Part model, mm, in its own coordinate system. Face numbers are marked on the shaded views. Coordinates: 2 decimals unless noted, no trailing zeros. Loops run counter-clockwise (first coordinate to the right, second up) from the corner with the lowest first, then second, coordinate; pieces in that order, holes last. Notation, with made-up numbers: M 81.5,6 L 116.5,6 A16 cw 116.5,29 Z; hole C 23.25,-29 d1. An arc over 180 degrees is marked long. Use a Markdown table: item, result. Add a question column.
1) Band-saw the part on C-C (x = 224.5). List the corners of the cut face in (y, z), plus the area to 3 significant figures.
2) Wall check: probe 1 along Y at (x, z) = (26.5, -12.5); probe 2 along Y at (x, z) = (26.5, -9.25); probe 3 along Z at (x, y) = (249, 51.5). Give the ranges that are in metal, low to high. Write a range as from..to.
3) Band-saw the part on B-B (x = 65). List the corners of the cut face in (y, z).
4) Pull direction Y, two halves, no side cores. Call the marked faces 1 and 2: released by +Y, released by -Y, zero draft, split by the parting line, or undercut.
5) Pin check, flat tips, straight feed: pin 1 Ø0.8 at (x, z) = (112.5, -14.5) entering from -Y; pin 2 Ø0.8 at (x, z) = (140, -14.5) entering from +Y; pin 3 Ø1.4 at (x, y) = (165, 69) entering from -Z; pin 4 Ø1 at (y, z) = (60, -11.5) entering from -X. Stop position of each tip, or through.
6) Band-saw the part on A-A (z = -11.75). List the corners of the cut face in (x, y), plus the area to 3 significant figures.
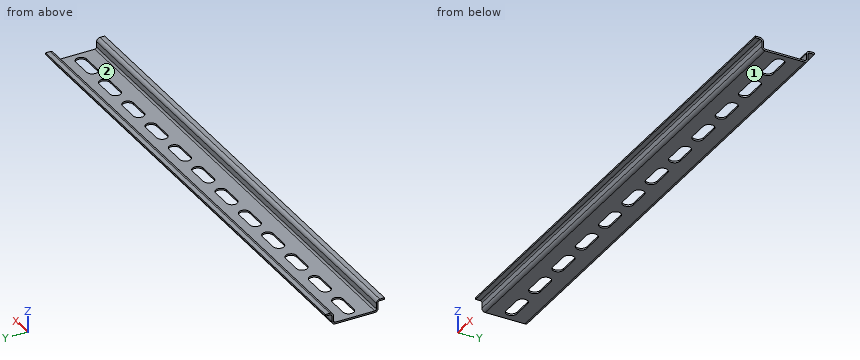
Autodesk Inventor part; units mm, degrees
ref_plane "YZ Plane" through (0, 0, 0) normal (1, 0, 0) x (0, 1, 0)
ref_plane "XZ Plane" through (0, 0, 0) normal (0, 1, 0) x (-1, 0, 0)
ref_plane "XY Plane" through (0, 0, 0) normal (0, 0, 1) x (1, 0, 0)
sketch "Sketch1" plane through (0, 0, 0) normal (1, 0, 0) x (0, 1, 0)
  line L0 (41.284, -14.8819) -> (64.684, -14.8819)
  line L1 (64.684, -13.8819) -> (41.284, -13.8819)
  line L2 (67.684, -8.5819) -> (70.484, -8.5819)
  line L3 (70.484, -8.5819) -> (70.484, -7.5819)
  line L4 (70.484, -7.5819) -> (67.684, -7.5819)
  line L5 (-1817770.1114, -20.3632) -> (-1817770.1114, -8.5819)
  line L6 (38.284, -7.5819) -> (35.484, -7.5819)
  line L7 (35.484, -7.5819) -> (35.484, -8.5819)
  line L8 (35.484, -8.5819) -> (38.284, -8.5819)
  line L9 (40.284, -9.5819) -> (40.284, -12.8819)
  arc A0 (67.684, -8.5819) -> (66.684, -9.5819) centre (67.684, -9.5819) ccw
  arc A1 (64.684, -13.8819) -> (65.684, -12.8819) centre (64.684, -12.8819) ccw
  arc A2 (40.284, -12.8819) -> (41.284, -13.8819) centre (41.284, -12.8819) ccw
  arc A3 (39.284, -9.5819) -> (38.284, -8.5819) centre (38.284, -9.5819) ccw
  arc A4 (40.284, -9.5819) -> (38.284, -7.5819) centre (38.284, -9.5819) ccw
  arc A5 (39.284, -12.8819) -> (41.284, -14.8819) centre (41.284, -12.8819) ccw
  line L10 (39.284, -9.5819) -> (39.284, -12.8819)
  arc A6 (67.684, -7.5819) -> (65.684, -9.5819) centre (67.684, -9.5819) ccw
  arc A7 (64.684, -14.8819) -> (66.684, -12.8819) centre (64.684, -12.8819) ccw
  line L11 (66.684, -9.5819) -> (66.684, -12.8819)
  line L12 (65.684, -9.5819) -> (65.684, -12.8819)
  line L13 (52.984, -4.8951) -> (52.984, -40.6352) construction
  line L14 (-285.558, -25.9225) -> (179.442, -25.9225)
  line L15 (179.442, -25.9225) -> (179.442, -22.9225)
  line L16 (-285.558, -22.9225) -> (179.442, -22.9225)
  line L17 (-285.558, -25.9225) -> (-285.558, -22.9225)
  point P0 (0, 0)
  point P1 (40.284, -11.2319)
  dimension "d0" = 1
  dimension "d1" = 1
  dimension "d5" = 35
  dimension "d8" = 7.3
  dimension "d9" = 1
  dimension "d10" = 1
  dimension "d11" = 2
  dimension "d12" = 2
  dimension "d13" = 12.7
  dimension "d15" = 12.7
  dimension "d16" = 4.8
  dimension "d17" = 4.8
  dimension "d20" = 1
  dimension "d21" = 1
  dimension "d22" = 2
extrude "Extrusion1" add sketch "Sketch1" along normal blind 300 contours A5 L10 A3 L8 L7 L6 A4 L9 A2 L1 A1 L12 A6 L4 L3 L2 A0 L11 A7 L0
sketch "Sketch2" plane through (0, 41.284, -13.8819) normal (0, 0, 1) x (1, 0, 0)
  line L0 (3.6, 11.7) -> (21.6, 11.7) construction
  line L1 (6.8, 8.5) -> (18.4, 8.5)
  line L2 (18.4, 14.9) -> (6.8, 14.9)
  arc A0 (6.8, 14.9) -> (6.8, 8.5) centre (6.8, 11.7) ccw
  arc A1 (18.4, 8.5) -> (18.4, 14.9) centre (18.4, 11.7) ccw
  line L3 (0, 29.2) -> (300, 29.2)
  line L4 (0, -5.8) -> (300, -5.8)
  line L5 (0, 23.4) -> (0, 0)
  arc A2 (31.8, 14.9) -> (31.8, 8.5) centre (31.8, 11.7) ccw
  line L6 (31.8, 8.5) -> (43.4, 8.5)
  arc A3 (43.4, 8.5) -> (43.4, 14.9) centre (43.4, 11.7) ccw
  line L7 (43.4, 14.9) -> (31.8, 14.9)
  arc A4 (56.8, 14.9) -> (56.8, 8.5) centre (56.8, 11.7) ccw
  line L8 (56.8, 8.5) -> (68.4, 8.5)
  arc A5 (68.4, 8.5) -> (68.4, 14.9) centre (68.4, 11.7) ccw
  line L9 (68.4, 14.9) -> (56.8, 14.9)
  arc A6 (81.8, 14.9) -> (81.8, 8.5) centre (81.8, 11.7) ccw
  line L10 (81.8, 8.5) -> (93.4, 8.5)
  arc A7 (93.4, 8.5) -> (93.4, 14.9) centre (93.4, 11.7) ccw
  line L11 (93.4, 14.9) -> (81.8, 14.9)
  arc A8 (106.8, 14.9) -> (106.8, 8.5) centre (106.8, 11.7) ccw
  line L12 (106.8, 8.5) -> (118.4, 8.5)
  arc A9 (118.4, 8.5) -> (118.4, 14.9) centre (118.4, 11.7) ccw
  line L13 (118.4, 14.9) -> (106.8, 14.9)
  arc A10 (131.8, 14.9) -> (131.8, 8.5) centre (131.8, 11.7) ccw
  line L14 (131.8, 8.5) -> (143.4, 8.5)
  arc A11 (143.4, 8.5) -> (143.4, 14.9) centre (143.4, 11.7) ccw
  line L15 (143.4, 14.9) -> (131.8, 14.9)
  arc A12 (156.8, 14.9) -> (156.8, 8.5) centre (156.8, 11.7) ccw
  line L16 (156.8, 8.5) -> (168.4, 8.5)
  arc A13 (168.4, 8.5) -> (168.4, 14.9) centre (168.4, 11.7) ccw
  line L17 (168.4, 14.9) -> (156.8, 14.9)
  arc A14 (181.8, 14.9) -> (181.8, 8.5) centre (181.8, 11.7) ccw
  line L18 (181.8, 8.5) -> (193.4, 8.5)
  arc A15 (193.4, 8.5) -> (193.4, 14.9) centre (193.4, 11.7) ccw
  line L19 (193.4, 14.9) -> (181.8, 14.9)
  line L20 (0, 0) -> (300, 0)
  line L21 (0, 24.4) -> (300, 24.4)
  line L22 (0, -1) -> (300, -1)
  arc A16 (206.8, 14.9) -> (206.8, 8.5) centre (206.8, 11.7) ccw
  line L23 (218.4, 14.9) -> (206.8, 14.9)
  arc A17 (218.4, 8.5) -> (218.4, 14.9) centre (218.4, 11.7) ccw
  line L24 (206.8, 8.5) -> (218.4, 8.5)
  arc A18 (231.8, 14.9) -> (231.8, 8.5) centre (231.8, 11.7) ccw
  line L25 (243.4, 14.9) -> (231.8, 14.9)
  arc A19 (243.4, 8.5) -> (243.4, 14.9) centre (243.4, 11.7) ccw
  line L26 (231.8, 8.5) -> (243.4, 8.5)
  arc A20 (256.8, 14.9) -> (256.8, 8.5) centre (256.8, 11.7) ccw
  line L27 (268.4, 14.9) -> (256.8, 14.9)
  arc A21 (268.4, 8.5) -> (268.4, 14.9) centre (268.4, 11.7) ccw
  line L28 (256.8, 8.5) -> (268.4, 8.5)
  arc A22 (281.8, 14.9) -> (281.8, 8.5) centre (281.8, 11.7) ccw
  line L29 (293.4, 14.9) -> (281.8, 14.9)
  arc A23 (293.4, 8.5) -> (293.4, 14.9) centre (293.4, 11.7) ccw
  line L30 (281.8, 8.5) -> (293.4, 8.5)
  point P0 (0, -41.284)
  point P1 (12.6, 11.7)
  point P2 (28.6, 11.7)
  point P3 (46.6, 11.7)
  point P4 (53.6, 11.7)
  point P5 (71.6, 11.7)
  point P6 (78.6, 11.7)
  point P7 (96.6, 11.7)
  point P8 (103.6, 11.7)
  point P9 (121.6, 11.7)
  point P10 (128.6, 11.7)
  point P11 (146.6, 11.7)
  point P12 (153.6, 11.7)
  point P13 (171.6, 11.7)
  point P14 (178.6, 11.7)
  point P15 (196.6, 11.7)
  point P16 (28.6, 11.7)
  point P17 (203.6, 11.7)
  point P18 (221.6, 11.7)
  point P19 (228.6, 11.7)
  point P20 (246.6, 11.7)
  point P21 (253.6, 11.7)
  point P22 (271.6, 11.7)
  point P23 (278.6, 11.7)
  point P24 (296.6, 11.7)
  dimension "d26" = 18
  dimension "d33" = 25
  dimension "d46" = 3.6
  dimension "d47" = 17.5
  dimension "d48" = 17.5
  dimension "d51" = 25
extrude "Extrusion2" cut sketch "Sketch2" against normal blind 25
sketch "Sketch3" plane through (0, 41.284, -13.8819) normal (0, 0, 1) x (1, 0, 0)
  line L0 (110, 34.2) -> (302, 34.2)
  line L1 (302, 34.2) -> (302, -10.8)
  line L2 (302, -10.8) -> (110, -10.8)
  line L3 (110, -10.8) -> (110, 34.2)
  line L4 (0, 23.4) -> (0, 0)
  line L5 (300, 23.4) -> (300, 0)
  line L6 (0, -5.8) -> (300, -5.8)
  line L7 (0, 29.2) -> (300, 29.2)
  point P0 (0, -41.284)
  dimension "d56" = 110
  dimension "d57" = 2
  dimension "d58" = 5
  dimension "d59" = 5
equation "\"d39\" = d33"
properties part number "DIN-rail"
Entries:
| question | item | result |
|---|---|---|
| 1 | outline | M 35.48,-8.58 L 38.28,-8.58 A1 cw 39.28,-9.58 L 39.28,-12.88 A2 ccw 41.28,-14.88 L 64.68,-14.88 A2 ccw 66.68,-12.88 L 66.68,-9.58 A1 cw 67.68,-8.58 L 70.48,-8.58 L 70.48,-7.58 L 67.68,-7.58 A2 ccw 65.68,-9.58 L 65.68,-12.88 A1 cw 64.68,-13.88 L 41.28,-13.88 A1 cw 40.28,-12.88 L 40.28,-9.58 A2 ccw 38.28,-7.58 L 35.48,-7.58 Z |
| 1 | area | 45.0 mm2 |
| 2 | probe 1 | 39.28..40.28, 65.68..66.68 |
| 2 | probe 2 | 39.23..40.26, 65.71..66.74 |
| 2 | probe 3 | -14.88..-13.88 |
| 3 | outline | M 35.48,-8.58 L 38.28,-8.58 A1 cw 39.28,-9.58 L 39.28,-12.88 A2 ccw 41.28,-14.88 L 49.78,-14.88 L 49.78,-13.88 L 41.28,-13.88 A1 cw 40.28,-12.88 L 40.28,-9.58 A2 ccw 38.28,-7.58 L 35.48,-7.58 Z; M 56.18,-14.88 L 64.68,-14.88 A2 ccw 66.68,-12.88 L 66.68,-9.58 A1 cw 67.68,-8.58 L 70.48,-8.58 L 70.48,-7.58 L 67.68,-7.58 A2 ccw 65.68,-9.58 L 65.68,-12.88 A1 cw 64.68,-13.88 L 56.18,-13.88 Z |
| 4 | face 1 | zero draft |
| 4 | face 2 | undercut |
| 5 | pin 1 | y = 39.7 |
| 5 | pin 2 | y = 66.27 |
| 5 | pin 3 | z = -8.58 |
| 5 | pin 4 | through |
| 6 | outline | M 0,39.28 L 300,39.28 L 300,40.28 L 0,40.28 Z; M 0,65.68 L 300,65.68 L 300,66.68 L 0,66.68 Z |
| 6 | area | 600 mm2 |
